Geometry check sheet. Reference: the model listing, model coordinates, mm. Round coordinates to 2 decimals unless told otherwise and drop trailing zeros. Order: outer loops, then holes, each group sorted by start corner. A loop starts at its lowest first (then second) coordinate and runs counter-clockwise, first axis right, second up.
```python
from build123d import *

# Parameters (mm, degrees)
SKETCH1_W                 = 203.2
SKETCH1_H                 = 25.4
BOSS_EXTRUDE1_DEPTH       = 9.525
F_8_CLEARANCE_HOLE1_D     = 4.4958
F_8_CLEARANCE_HOLE1_DEPTH = 25.4
F_8_CLEARANCE_HOLE1_TIP   = 1.350674586
SKETCH5_R                 = 3.1623
CUT_EXTRUDE1_DEPTH        = 9.525
F_8_CLEARANCE_HOLE2_D     = 4.4958
F_8_CLEARANCE_HOLE2_DEPTH = 19.05
F_8_CLEARANCE_HOLE2_TIP   = 1.350674586
CUT_EXTRUDE2_DEPTH        = 10.525


with BuildPart() as part:
    # Sketch1 → Boss-Extrude1 (new body)
    with BuildSketch(Plane.XY):
        with Locations((-101.6, 12.7)):
            Rectangle(SKETCH1_W, SKETCH1_H)
    extrude(amount=BOSS_EXTRUDE1_DEPTH)

    # #8 Clearance Hole1
    with Locations(Plane.XY.offset(9.525)):
        with Locations((-4.7625, 6.35), (-4.7625, 19.05)):
            Hole(F_8_CLEARANCE_HOLE1_D / 2, depth=F_8_CLEARANCE_HOLE1_DEPTH)
            with Locations((0, 0, -(F_8_CLEARANCE_HOLE1_DEPTH + F_8_CLEARANCE_HOLE1_TIP / 2))):  # 118° drill point
                Cone(0, F_8_CLEARANCE_HOLE1_D / 2, F_8_CLEARANCE_HOLE1_TIP, mode=Mode.SUBTRACT)

    # Sketch5 → Cut-Extrude1 (cut)
    with BuildSketch(Plane.XY.offset(9.525)):
        with Locations((-184.15, 12.7)):
            Circle(SKETCH5_R)
    extrude(amount=-CUT_EXTRUDE1_DEPTH, mode=Mode.SUBTRACT)

    # #8 Clearance Hole2
    with Locations(Plane.XY.offset(9.525)):
        with Locations((-120.65, 12.7)):
            Hole(F_8_CLEARANCE_HOLE2_D / 2, depth=F_8_CLEARANCE_HOLE2_DEPTH)
            with Locations((0, 0, -(F_8_CLEARANCE_HOLE2_DEPTH + F_8_CLEARANCE_HOLE2_TIP / 2))):  # 118° drill point
                Cone(0, F_8_CLEARANCE_HOLE2_D / 2, F_8_CLEARANCE_HOLE2_TIP, mode=Mode.SUBTRACT)

    # Sketch10 → Cut-Extrude2 (cut, through all)
    with BuildSketch(Plane.XY.offset(9.525)):
        with BuildLine():
            Line((-190.5, 25.4), (-203.2, 25.4))
            Line((-203.2, 25.4), (-203.2, 12.7))
            ThreePointArc((-203.2, 12.7), (-199.480256121, 21.680256121), (-190.5, 25.4))
        make_face()
        with BuildLine():
            ThreePointArc((-190.5, 0), (-199.480256121, 3.719743879), (-203.2, 12.7))
            Line((-203.2, 12.7), (-203.2, 0))
            Line((-203.2, 0), (-190.5, 0))
        make_face()
    extrude(amount=-CUT_EXTRUDE2_DEPTH, mode=Mode.SUBTRACT)


solid = part.part
```
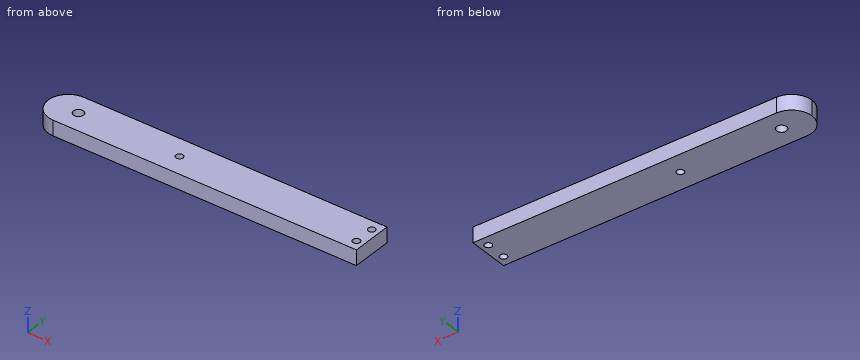
(1) Sectioned sample at B-B, the plane z = 6.25. Record the cut outline in (x, y), and give its area (3 significant figures).
Returned:
outline: (-190.5, 0) - (0, 0) - (0, 25.4) - (-190.5, 25.4) arc R12.7 ccw to start; hole circle Ø6.32 at (-184.15, 12.7); hole circle Ø4.5 at (-120.65, 12.7); hole circle Ø4.5 at (-4.76, 6.35); hole circle Ø4.5 at (-4.76, 19.05)
area: 5,010 mm2
(2) Depth check by flat-ended pin: P1, Ø5, axis at x = -120.65, y = 12.7, coming from the +Z side (3 decimals); P2, Ø2.5, axis at x = -4.76, y = 19.05, coming from the -Z side; P3, Ø1, axis at y = 8.5, z = 6.5, coming from the -X side. Enter the tip coordinate at first touch or a pass-through.
Returned:
P1: stops at z = 9.525
P2: passes through
P3: stops at x = -202.65
(3) Sectioned sample at C-C, the plane y = 19.05. Record the cut outline in (x, z) (3 decimals), and give its area (3 significant figures).
Returned:
outline: (-201.499, 0) - (-7.01, 0) - (-7.01, 9.525) - (-201.499, 9.525) - close; (-2.515, 0) - (0, 0) - (0, 9.525) - (-2.515, 9.525) - close
area: 1,880 mm2
(4) Sectioned sample at A-A, the plane x = -184.15. Record the cut outline in (y, z) (3 decimals).
Returned:
outline: (0, 0) - (9.538, 0) - (9.538, 9.525) - (0, 9.525) - close; (15.862, 0) - (25.4, 0) - (25.4, 9.525) - (15.862, 9.525) - close
(5) Material ranges on line 1 (Y direction, x = -120.65, z = 7.25); line 2 (X direction, y = 8, z = 3); line 3 (Y direction, x = -185.5, z = 5.25), recorded low to high.
Returned:
line 1: y = 0 to 10.45, 14.95 to 25.4
line 2: x = -202.3 to -6.29, -3.24 to 0
line 3: y = 0 to 9.84, 15.56 to 25.4
